Check sheet for the modelled part. Datum: model origin and axes. Units: mm. Coordinates: 2 decimals unless noted, no trailing zeros. Write each loop counter-clockwise with the first axis right and the second up, starting at its lowest first coordinate (ties: lowest second). Pieces come first, ordered by that corner, then holes. Notation, with made-up numbers: (-8, 21.5) - (40, 21.5) arc R27 ccw to (40, 50.5) - close; hole circle Ø4 at (-2.5, 73). An arc over 180 degrees is marked (long way). Write each question's results on one line, items separated by ' | '.
from build123d import *

# Parameters (mm, degrees)
SKETCH_1_R        = 2.5
BODY_DEPTH        = 406.5
CHAMFEREDGES_SIZE = 0.5
SKETCH2_W         = 28.630475487
SKETCH2_H         = 2.50986962
SKETCH2_W_2       = 28
SKETCH2_H_2       = 1.942146438
FIRSTSLOTS_DEPTH  = 407.515374863
CIRPATTERN1_COUNT = 2
CIRPATTERN1_ANGLE = 90


with BuildPart() as part:
    # Эскиз1 → Body (new body)
    with BuildSketch(Plane.XY):
        with Locations(Location((0, 0, 0), (0, 0, 180))):
            Circle(SKETCH_1_R)
    extrude(amount=BODY_DEPTH)

    # ChamferEdges
    chamferedges_edges = [part.edges().sort_by_distance(p)[0] for p in [
        (2.5, 0, 0),
        (2.5, 0, 406.5),
    ]]
    chamfer(chamferedges_edges, length=CHAMFEREDGES_SIZE)

    # Sketch2 → FirstSlots (cut, symmetric)
    with BuildSketch(Plane(origin=(0, 0, 0), x_dir=(0, 0, -1), z_dir=(1, 0, 0))):
        with Locations((-13.684762257, 2.75493481)):
            Rectangle(SKETCH2_W, SKETCH2_H)
        with Locations((-398.5, 2.471073219)):
            Rectangle(SKETCH2_W_2, SKETCH2_H_2)
    firstslots = extrude(amount=FIRSTSLOTS_DEPTH, both=True, mode=Mode.SUBTRACT)

    # CirPattern1: FirstSlots ×2 about axis
    cirpattern1_axis = Axis((0, 0, 406.5), (0, 0, 1))
    for i in range(1, CIRPATTERN1_COUNT):
        add(firstslots.rotate(cirpattern1_axis, i * CIRPATTERN1_ANGLE / (CIRPATTERN1_COUNT - 1)), mode=Mode.SUBTRACT)


solid = part.part
1. Material ranges on L1, parallel to X at y = 0.1, z = 323; L2, parallel to Y at x = -1.45, z = 257.5; L3, parallel to Z at x = -0.35, y = 2.15, recorded low to high. Write a range as [from, to].
Values follow:
L1: x = [-2.5, 2.5] | L2: y = [-2.04, 2.04] | L3: z = [28, 384.5]
2. Sectioned sample at B-B (y = 0). Record the cut outline in (x, z).
Values follow:
outline: (-2.5, 28) - (-1.5, 28) - (-1.5, 0) - (2, 0) - (2.5, 0.5) - (2.5, 406) - (2, 406.5) - (-1.5, 406.5) - (-1.5, 384.5) - (-2.5, 384.5) - close
3. Sectioned sample at A-A (x = 0). Record the cut outline in (y, z).
Values follow:
outline: (-2.5, 0.5) - (-2, 0) - (1.5, 0) - (1.5, 28) - (2.5, 28) - (2.5, 384.5) - (1.5, 384.5) - (1.5, 406.5) - (-2, 406.5) - (-2.5, 406) - close
4. Go/stop test with flat-tipped pins: pin 1 (2 mm diameter, centred on x = 0.5, y = 0, fed in from -Z); pin 2 (1.5 mm diameter, centred on x = -1, z = 135.5, fed in from +Y); pin 3 (1 mm diameter, centred on x = 1.5, z = 302, fed in from -Y). Record where each tip stops, or that it passes through.
Values follow:
pin 1: stops at z = 0 | pin 2: stops at y = 2.49 | pin 3: stops at y = -2.29
5. Sectioned sample at C-C (z = 255.5). Record the cut outline in (x, y).
Values follow:
outline: circle Ø5 at (0, 0)
